```python
from build123d import *

# Parameters (mm, degrees)
SKETCH1_W           = 5
SKETCH1_H           = 16.5
SKETCH1_W_2         = 12
SKETCH1_H_2         = 5
SKETCH1_H_3         = 4
SKETCH1_W_3         = 24.5
SKETCH1_W_4         = 4
BOSS_EXTRUDE1_DEPTH = 4
FILLET1_R           = 10
FILLET2_R           = 1


with BuildPart() as part:
    # Sketch1 → Boss-Extrude1 (new body)
    # profile 1 of 16: a face of its own
    with BuildSketch(Plane(origin=(0, 0, 0), x_dir=(1, 0, 0), z_dir=(0, 1, 0))):
        Polygon((-78, 42.5), (-58.890996312, 42.5), (-50.5, 32.5), (-50.5, -32.5), (50.5, -32.5), (50.5, 32.5), (62.417535926, 42.5), (78, 42.5), (78, -47.5), (-78, -47.5), align=None)
        Polygon((-74, 39.5), (-61.595326576, 39.5), (-59.688086754, 37.22704009), (-74, -32.5), align=None, mode=Mode.SUBTRACT)
        Polygon((-56.407239822, 33.317078972), (-54.5, 31.044119063), (-54.5, -32.5), (-69.916608972, -32.5), align=None, mode=Mode.SUBTRACT)
        Polygon((-74, -36.5), (-74, -43.5), (-45.997033515, -43.5), align=None, mode=Mode.SUBTRACT)
        Polygon((-57.50593297, -36.5), (-7.972135955, -36.5), (-4.472135955, -43.5), (-29.502966485, -43.5), align=None, mode=Mode.SUBTRACT)
        Polygon((3.5, -36.5), (-3.5, -36.5), (0, -43.5), align=None, mode=Mode.SUBTRACT)
        Polygon((4.472135955, -43.5), (29.502966485, -43.5), (57.50593297, -36.5), (7.972135955, -36.5), align=None, mode=Mode.SUBTRACT)
        Polygon((74, -43.5), (45.997033515, -43.5), (74, -36.5), align=None, mode=Mode.SUBTRACT)
        Polygon((54.5, -32.5), (69.916608972, -32.5), (56.407239822, 33.317078972), (54.5, 31.044119063), align=None, mode=Mode.SUBTRACT)
        Polygon((59.688086754, 37.22704009), (74, -32.5), (74, 39.5), (61.595326576, 39.5), align=None, mode=Mode.SUBTRACT)
    # profile 2 of 16: a face of its own
    with BuildSketch(Plane(origin=(0, 0, 0), x_dir=(1, 0, 0), z_dir=(0, 1, 0))):
        with Locations((80.5, 31.25)):
            Rectangle(SKETCH1_W, SKETCH1_H)
    # profile 3 of 16: a face of its own
    with BuildSketch(Plane(origin=(0, 0, 0), x_dir=(1, 0, 0), z_dir=(0, 1, 0))):
        with Locations((80.5, -36.25)):
            Rectangle(SKETCH1_W, SKETCH1_H)
    # profile 4 of 16: a face of its own
    with BuildSketch(Plane(origin=(0, 0, 0), x_dir=(1, 0, 0), z_dir=(0, 1, 0))):
        with Locations((0, -50)):
            Rectangle(SKETCH1_W_2, SKETCH1_H_2)
    # profile 5 of 16: a face of its own
    with BuildSketch(Plane(origin=(0, 0, 0), x_dir=(1, 0, 0), z_dir=(0, 1, 0))):
        with Locations((80.5, 18)):
            Rectangle(SKETCH1_W, SKETCH1_H_3)
    # profile 6 of 16: a face of its own
    with BuildSketch(Plane(origin=(0, 0, 0), x_dir=(1, 0, 0), z_dir=(0, 1, 0))):
        with Locations((80.5, -23)):
            Rectangle(SKETCH1_W, SKETCH1_H_3)
    # profile 7 of 16: a face of its own
    with BuildSketch(Plane(origin=(0, 0, 0), x_dir=(1, 0, 0), z_dir=(0, 1, 0))):
        with Locations((37.75, -50)):
            Rectangle(SKETCH1_W_3, SKETCH1_H_2)
    # profile 8 of 16: a face of its own
    with BuildSketch(Plane(origin=(0, 0, 0), x_dir=(1, 0, 0), z_dir=(0, 1, 0))):
        with Locations((55, -50)):
            Rectangle(SKETCH1_W_4, SKETCH1_H_2)
    # profile 9 of 16: a face of its own
    with BuildSketch(Plane(origin=(0, 0, 0), x_dir=(1, 0, 0), z_dir=(0, 1, 0))):
        with Locations((20.5, -50)):
            Rectangle(SKETCH1_W_4, SKETCH1_H_2)
    # profile 10 of 16: a face of its own
    with BuildSketch(Plane(origin=(0, 0, 0), x_dir=(1, 0, 0), z_dir=(0, 1, 0))):
        with Locations((-20.5, -50)):
            Rectangle(SKETCH1_W_4, SKETCH1_H_2)
    # profile 11 of 16: a face of its own
    with BuildSketch(Plane(origin=(0, 0, 0), x_dir=(1, 0, 0), z_dir=(0, 1, 0))):
        with Locations((-37.75, -50)):
            Rectangle(SKETCH1_W_3, SKETCH1_H_2)
    # profile 12 of 16: a face of its own
    with BuildSketch(Plane(origin=(0, 0, 0), x_dir=(1, 0, 0), z_dir=(0, 1, 0))):
        with Locations((-55, -50)):
            Rectangle(SKETCH1_W_4, SKETCH1_H_2)
    # profile 13 of 16: a face of its own
    with BuildSketch(Plane(origin=(0, 0, 0), x_dir=(1, 0, 0), z_dir=(0, 1, 0))):
        with Locations((-80.5, -36.25)):
            Rectangle(SKETCH1_W, SKETCH1_H)
    # profile 14 of 16: a face of its own
    with BuildSketch(Plane(origin=(0, 0, 0), x_dir=(1, 0, 0), z_dir=(0, 1, 0))):
        with Locations((-80.5, -23)):
            Rectangle(SKETCH1_W, SKETCH1_H_3)
    # profile 15 of 16: a face of its own
    with BuildSketch(Plane(origin=(0, 0, 0), x_dir=(1, 0, 0), z_dir=(0, 1, 0))):
        with Locations((-80.5, 18)):
            Rectangle(SKETCH1_W, SKETCH1_H_3)
    # profile 16 of 16: a face of its own
    with BuildSketch(Plane(origin=(0, 0, 0), x_dir=(1, 0, 0), z_dir=(0, 1, 0))):
        with Locations((-80.5, 31.25)):
            Rectangle(SKETCH1_W, SKETCH1_H)
    extrude(amount=BOSS_EXTRUDE1_DEPTH)

    # Fillet1
    fillet1_edges = [part.edges().sort_by_distance(p)[0] for p in [
        (-58.890996312, 2, -42.5),
        (-50.5, 2, -32.5),
        (-50.5, 2, 32.5),
        (50.5, 2, 32.5),
        (50.5, 2, -32.5),
        (62.417535926, 2, -42.5),
    ]]
    fillet(fillet1_edges, radius=FILLET1_R)

    # Fillet2
    fillet2_edges = [part.edges().sort_by_distance(p)[0] for p in [
        (74, 2, 43.5),
        (74, 2, 36.5),
        (45.997033515, 2, 43.5),
        (-3.5, 2, 36.5),
        (0, 2, 43.5),
        (3.5, 2, 36.5),
        (-4.472135955, 2, 43.5),
        (-7.972135955, 2, 36.5),
        (-57.50593297, 2, 36.5),
        (-29.502966485, 2, 43.5),
        (-54.5, 2, 32.5),
        (-54.5, 2, -31.044119063),
        (-56.407239822, 2, -33.317078972),
        (-69.916608972, 2, 32.5),
        (-59.688086754, 2, -37.22704009),
        (-61.595326576, 2, -39.5),
        (-74, 2, -39.5),
        (-74, 2, 32.5),
        (-74, 2, 36.5),
        (-74, 2, 43.5),
        (-45.997033515, 2, 43.5),
        (57.50593297, 2, 36.5),
        (7.972135955, 2, 36.5),
        (4.472135955, 2, 43.5),
        (29.502966485, 2, 43.5),
        (56.407239822, 2, -33.317078972),
        (54.5, 2, -31.044119063),
        (54.5, 2, 32.5),
        (69.916608972, 2, 32.5),
        (74, 2, -39.5),
        (61.595326576, 2, -39.5),
        (59.688086754, 2, -37.22704009),
        (74, 2, 32.5),
    ]]
    fillet(fillet2_edges, radius=FILLET2_R)


solid = part.part
```
CAD build for the part. Positions are in the model's coordinates, mm. A direction names the side the tool comes from. Coordinates: 2 decimals unless noted, no trailing zeros. Loops run counter-clockwise (first coordinate to the right, second up) from the corner with the lowest first, then second, coordinate; pieces in that order, holes last. Notation, with made-up numbers: (9.25, 21.5) - (63.25, 21.5) arc R29 ccw to (63.25, 44.5) - close; hole circle Ø2 at (86.5, 63). An arc over 180 degrees is marked (long way). Use CSV: the item, a comma, the result in double quotes. Start each with the question number.
Q1. 3-axis set-ups, long thin cutter, end or side, ignore diameter. For faces 4 (the flat face through (80, 2, 28)), 5 (the flat face through (-81, 2, -16)), 6 (the flat face through (39.5, 2, 41)), 7 (the flat face through (12, 2, 47.5)), 8 (the flat face through (-1, 2, 32.5)): which of +Z, -Z, +X, -X, +Y, -Y reach the whole face in a straight line?
Q2. Drop flat-ended pins along their axis: P1, Ø1.2, axis at x = -14.5, y = 1, coming from the +Z side; P2, Ø2, axis at y = 1, z = 51, coming from the +X side; P3, Ø1, axis at y = 1, z = 15.5, coming from the +X side. Give the stop position or say it passes through.
Q3. Cut at C-C, the plane x = 42.5. List the corners of the cut face in (y, z), then the cut area to 3 significant figures.
Q4. Cut at A-A, the plane x = -15.5. List the corners of the cut face in (y, z).
Q5. Cut at B-B, the plane z = 19. List the corners of the cut face in (x, y).
Q6. Two-plate mould, pull along Z, no slides. Class faces 1 (the flat face through (20, 2, 52.5)), 2 (the flat face through (-74, 2, -7)), 3 (the flat face through (78, 2, -41)): +Z half, -Z half, draft (parallel to the pull), parting line (faces both ways), or undercut.
Q7. Probe probe 1 along Z at (x, y) = (-9.5, 1.5); probe 2 along X at (y, z) = (1.1, 30); probe 3 along X at (y, z) = (1.6, 26). List the from-to ranges inside material, lowest first. Write a range as from..to.
Q8. Cut at D-D, the plane y = 2.9. State how many separate pieces and enclosed holes the cut face has, then the cut area to 3 significant figures.
Here are the results:
1,face 4,"+X, +Y, -Y"
1,face 5,"-X, +Y, -Y"
1,face 6,"+Y, -Y"
1,face 7,"+Z, +Y, -Y"
1,face 8,"-Z, +Y, -Y"
2,P1,"z = 47.5"
2,P2,"x = 57"
2,P3,"x = 78"
3,outline,"(0, 32.3) - (4, 32.3) - (4, 36.5) - (0, 36.5) - close; (0, 40.25) - (4, 40.25) - (4, 52.5) - (0, 52.5) - close"
3,area,"65.8 mm2"
4,outline,"(0, 32.5) - (4, 32.5) - (4, 36.5) - (0, 36.5) - close; (0, 43.5) - (4, 43.5) - (4, 47.5) - (0, 47.5) - close"
5,outline,"(-78, 0) - (-74, 0) - (-74, 4) - (-78, 4) - close; (-71.23, 0) - (-67.15, 0) - (-67.15, 4) - (-71.23, 4) - close; (-54.5, 0) - (-50.5, 0) - (-50.5, 4) - (-54.5, 4) - close; (50.5, 0) - (54.5, 0) - (54.5, 4) - (50.5, 4) - close; (67.15, 0) - (71.23, 0) - (71.23, 4) - (67.15, 4) - close; (74, 0) - (78, 0) - (78, 4) - (74, 4) - close"
6,face 1,"+Z half"
6,face 2,"undercut"
6,face 3,"draft"
7,probe 1,"32.5..36.5, 43.5..47.5"
7,probe 2,"-83..-69.4, -54.5..-47.11, 47.11..54.5, 69.4..83"
7,probe 3,"-78..-68.58, -54.5..-49.87, 49.87..54.5, 68.58..78"
8,separate pieces,"1"
8,enclosed holes,"9"
8,area,"4,310 mm2"
